Can you work these out from the model? Positions are in its coordinate system, mm. A direction names the side the tool comes from. Give positions to 0.01 mm unless a question says otherwise; leave off trailing zeros. Order: outer loops, then holes, each group sorted by start corner. A loop starts at its lowest first (then second) coordinate and runs counter-clockwise, first axis right, second up. Notation, with made-up numbers: M 65.5,-19 L 103.5,-19 A3 ccw 103.5,-15 Z; hole C 41,45.25 d7. An arc over 180 degrees is marked long. Answer as a JSON object with one key per item and string values.
Autodesk Fusion 360 part; units mm, degrees
sketch "Sketch1" plane through (0, 0, 0) normal (0, 0, 1) x (1, 0, 0)
  line L0 (-27, -47.5) -> (27, -47.5)
  line L1 (27, -47.5) -> (27, 47.5)
  line L2 (27, 47.5) -> (-27, 47.5)
  line L3 (-27, 47.5) -> (-27, -47.5)
  line L4 (-27, -47.5) -> (27, 47.5) construction
  line L5 (27, -47.5) -> (-27, 47.5) construction
  dimension "d1" = 95
  dimension "d2" = 54
extrude "Extrude1" add sketch "Sketch1" along normal blind 11
sketch "Sketch2" plane through (0, 0, 11) normal (0, 0, 1) x (-1, 0, 0)
  line L0 (27, -47.5) -> (27, 47.5)
  line L1 (27, 47.5) -> (-27, 47.5)
  line L2 (-27, 47.5) -> (-27, -47.5)
  line L3 (-27, -47.5) -> (27, -47.5)
  line L4 (24.5, -45) -> (-24.5, -45)
  line L5 (-24.5, -45) -> (-24.5, 45)
  line L6 (-24.5, 45) -> (24.5, 45)
  line L7 (24.5, 45) -> (24.5, -45)
  line L8 (24.5, -45) -> (-24.5, 45) construction
  line L9 (-24.5, -45) -> (24.5, 45) construction
  dimension "d5" = 2.5
  dimension "d6" = 2.5
  dimension "d7" = 2.5
  dimension "d8" = 90
extrude "Extrude2" add sketch "Sketch2" along normal blind 5
extrude "Extrude3" cut 1 faces at (-8.1667, -15, 11) along direction (0, 0, -1) blind 5
sketch "Sketch3" plane through (0, 0, 6) normal (0, 0, 1) x (-1, 0, 0)
  line L0 (-24.5, 45) -> (-24.5, -45)
  line L1 (-24.5, -45) -> (24.5, -45)
  line L2 (24.5, -45) -> (24.5, 45)
  line L3 (24.5, 45) -> (-24.5, 45)
  line L4 (7.5, 45) -> (-7.5, 45)
  line L5 (-7.5, 45) -> (-7.5, -45)
  line L6 (-7.5, -45) -> (7.5, -45)
  line L7 (7.5, -45) -> (7.5, 45)
  line L8 (7.5, 45) -> (-7.5, -45) construction
  line L9 (-7.5, 45) -> (7.5, -45) construction
  dimension "d13" = 90
  dimension "d14" = 15
extrude "Extrude4" add sketch "Sketch3" along normal blind 8 contours L1 L3 L4 L5 L6 L7
sketch "Sketch4" plane through (0, 0, 14) normal (0, 0, 1) x (-1, 0, 0)
  line L0 (7.5, -45) -> (7.5, 45)
  line L1 (7.5, 45) -> (-7.5, 45)
  line L2 (-7.5, 45) -> (-7.5, -45)
  line L3 (-7.5, -45) -> (7.5, -45)
  line L4 (-6.5, 44.9) -> (6.5, 44.9)
  line L5 (6.5, 44.9) -> (6.5, -44.9)
  line L6 (6.5, -44.9) -> (-6.5, -44.9)
  line L7 (-6.5, -44.9) -> (-6.5, 44.9)
  line L8 (-6.5, 44.9) -> (6.5, -44.9) construction
  line L9 (6.5, 44.9) -> (-6.5, -44.9) construction
  dimension "d41" = 0.1
  dimension "d42" = 13
extrude "Extrude5" cut sketch "Sketch4" against normal blind 9 contours L4 L5 L6 L7
sketch "Sketch5" plane through (0, 0, 5) normal (0, 0, 1) x (-1, 0, 0)
  line L0 (-6.5, -44.9) -> (6.5, -44.9)
  line L1 (6.5, -44.9) -> (6.5, 44.9)
  line L2 (6.5, 44.9) -> (-6.5, 44.9)
  line L3 (-6.5, 44.9) -> (-6.5, -44.9)
  line L4 (-1.5, 36.5) -> (1.5, 36.5)
  line L5 (1.5, 36.5) -> (1.5, -36.5)
  line L6 (1.5, -36.5) -> (-1.5, -36.5)
  line L7 (-1.5, -36.5) -> (-1.5, 36.5)
  line L8 (-1.5, 36.5) -> (1.5, -36.5) construction
  line L9 (1.5, 36.5) -> (-1.5, -36.5) construction
  dimension "d21" = 3
  dimension "d22" = 73
extrude "Extrude6" cut sketch "Sketch5" against normal blind 5 contours L4 L5 L6 L7
sketch "Sketch6" plane through (0, 0, 16) normal (0, 0, 1) x (-1, 0, 0)
  line L0 (-24.5, 45) -> (24.5, 45)
  line L1 (24.5, 45) -> (24.5, -45)
  line L2 (24.5, -45) -> (-24.5, -45)
  line L3 (-24.5, -45) -> (-24.5, 45)
  line L4 (-27, -47.5) -> (27, -47.5)
  line L5 (27, -47.5) -> (27, 47.5)
  line L6 (27, 47.5) -> (-27, 47.5)
  line L7 (-27, 47.5) -> (-27, -47.5)
  line L8 (-25.5, -46) -> (25.5, -46)
  line L9 (25.5, -46) -> (25.5, 46)
  line L10 (25.5, 46) -> (-25.5, 46)
  line L11 (-25.5, 46) -> (-25.5, -46)
  line L12 (-25.5, -46) -> (25.5, 46) construction
  line L13 (25.5, -46) -> (-25.5, 46) construction
  dimension "d25" = 1.5
  dimension "d26" = 1.5
extrude "Extrude7" add sketch "Sketch6" along normal blind 5 contours L8 L9 L10 L11
sketch "Sketch7" plane through (0, 47.5, 0) normal (0, 1, 0) x (-1, 0, 0)
  line L0 (-27, 0) -> (27, 0)
  line L1 (27, 0) -> (27, 16)
  line L2 (27, 16) -> (-27, 16)
  line L3 (-27, 16) -> (-27, 0)
  circle A0 centre (14.9884, 9.9657) radius 5
  dimension "d29" = 10
extrude "Extrude8" add sketch "Sketch7" along normal blind 2 contours A0
fillet "Fillet1" radius 1 1 edges at (-10.3267, 49.5, 8.1576)
sketch "Sketch8" plane through (0, 49.5, 0) normal (0, 1, 0) x (-1, 0, 0)
  circle A0 centre (14.9884, 9.9657) radius 4
sketch "Sketch9" plane through (0, 49.5, 0) normal (0, 1, 0) x (-1, 0, 0)
  circle A0 centre (14.9884, 9.9657) radius 3
  point P0 (14.9884, 9.9657)
  dimension "d34" = 6
extrude "Extrude9" cut sketch "Sketch9" against normal blind 5
fillet "Fillet2" radius 2 4 edges at (-27, 47.5, 8) (27, 47.5, 8) (-27, -47.5, 8) (27, -47.5, 8)
fillet "Fillet3" radius 2 8 edges at (27, 0, 0) (26.4142, 46.9142, 0) (0, 47.5, 0) (-26.4142, 46.9142, 0) (-27, 0, 0) (-26.4142, -46.9142, 0) (0, -47.5, 0) (26.4142, -46.9142, 0)
1) Thinking about a two-plate mould opening in X: for faces 5 (the face through (0, 46, 18)), 6 (the face through (-1.5, -1, 3)), 7 (the face through (26.43, 0.64, 0.6)), which applies, pulls with the +X half, pulls with the -X half, needs draft (parallel to the pull), parting line crosses it, or undercut?
Results found:
{"face 5": "needs draft", "face 6": "undercut", "face 7": "pulls with the +X half"}
2) I want a section at B-B on y = 5.5. Write out the boundary of the cut face in (x, z).
Results found:
{"outline": "M -27,2 A2 ccw -25,0 L -1.5,0 L -1.5,5 L -6.5,5 L -6.5,14 L -7.5,14 L -7.5,6 L -24.5,6 L -24.5,21 L -25.5,21 L -25.5,16 L -27,16 Z; M 1.5,0 L 25,0 A2 ccw 27,2 L 27,16 L 25.5,16 L 25.5,21 L 24.5,21 L 24.5,6 L 7.5,6 L 7.5,14 L 6.5,14 L 6.5,5 L 1.5,5 Z"}
3) I need wall thicknesses on L1, parallel to X at y = 13, z = 13; L2, parallel to X at y = 19.5, z = 15.25; L3, parallel to Y at x = 11.5, z = 18.5. Which ranges of each line are inside material? Lowest first, please.
Results found:
{"L1": "x = -27 to -24.5, -7.5 to -6.5, 6.5 to 7.5, 24.5 to 27", "L2": "x = -27 to -24.5, 24.5 to 27", "L3": "y = -46 to -45, 45 to 46"}
4) I'm going to push flat-ended pins straight in: pin 1 Ø3.5 at (x, z) = (-14.99, 9.97) entering from +Y; pin 2 Ø2 at (x, z) = (1, 14) entering from +Y; pin 3 Ø16.5 at (x, y) = (3, 3.5) entering from +Z. Where does each tip first touch, or does it pass through?
Results found:
{"pin 1": "stops at y = -45", "pin 2": "stops at y = 47.5", "pin 3": "stops at z = 14"}
5) I want a section at A-A on z = 3.5. Write out the boundary of the cut face in (x, y), and give its area (3 significant figures).
Results found:
{"outline": "M -27,-45.5 A2 ccw -25,-47.5 L 25,-47.5 A2 ccw 27,-45.5 L 27,45.5 A2 ccw 25,47.5 L -25,47.5 A2 ccw -27,45.5 Z; hole M -1.5,-36.5 L 1.5,-36.5 L 1.5,36.5 L -1.5,36.5 Z", "area": "4,910 mm²"}
6) I want a section at C-C on y = 43. Write out the boundary of the cut face in (x, z), and give its area (3 significant figures).
Results found:
{"outline": "M -27,2 A2 ccw -25,0 L 25,0 A2 ccw 27,2 L 27,16 L 25.5,16 L 25.5,21 L 24.5,21 L 24.5,6 L 7.5,6 L 7.5,14 L 6.5,14 L 6.5,5 L -6.5,5 L -6.5,14 L -7.5,14 L -7.5,6 L -24.5,6 L -24.5,21 L -25.5,21 L -25.5,16 L -27,16 Z", "area": "385 mm²"}
7) I want a section at D-D on x = 21. Write out the boundary of the cut face in (y, z), and give its area (3 significant figures).
Results found:
{"outline": "M -47.5,2 A2 ccw -45.5,0 L 45.5,0 A2 ccw 47.5,2 L 47.5,16 L 46,16 L 46,21 L 45,21 L 45,6 L -45,6 L -45,21 L -46,21 L -46,16 L -47.5,16 Z", "area": "628 mm²"}
8) For faces 1 (the face through (-9.993, 47.993, 9.746)), 2 (the face through (0, -46, 18)), 3 (the face through (7, 0, 14)), 4 (the face through (-26.43, 46.9, 8.9)), which set-ups out of +Z, -Z, +X, -X, +Y, -Y let a thin tool reach every point of the face, with its end or its side?
Results found:
{"face 1": "+Y", "face 2": "+Z, +X, -X, -Y", "face 3": "+Z", "face 4": "+Z, -Z, -X, +Y"}
